```python
from build123d import *

# Parameters (mm, degrees)
FILLET1_R = 10


with BuildPart() as part:
    # Sketch1 → Revolve1 (revolve)
    with BuildSketch(Plane.XY, mode=Mode.PRIVATE) as revolve1_sk:
        Polygon((37.5, 42.257268448), (13.285767388, 0.316987298), (13.285767388, -0.683012702), (20.059447639, -25.962731552), (22.13, -25.962731552), (15.249019056, -0.282561065), (25.375644347, 17.257268448), (38.71, 17.257268448), (38.71, 42.257268448), align=None)
    revolve(revolve1_sk.sketch.rotate(Axis((0, 0, 0), (0, -1, 0)), 90), axis=Axis((0, 0, 0), (0, -1, 0)))

    # Fillet1
    fillet1_edges = [part.edges().sort_by_distance(p)[0] for p in [
        (0, 17.257268448, -25.375644347),
        (0, -0.282561065, -15.249019056),
    ]]
    fillet(fillet1_edges, radius=FILLET1_R)


solid = part.part
```
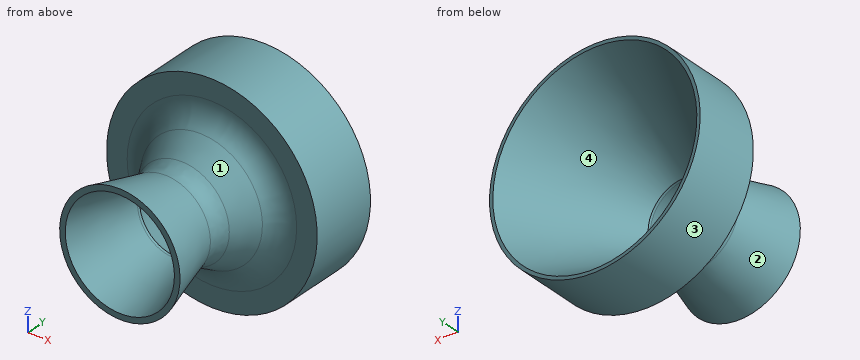
Input: part model. Units: mm. Frame: model coordinates. Face numbers are marked on the shaded views. Give positions to 0.01 mm unless a question says otherwise; leave off trailing zeros. Order: outer loops, then holes, each group sorted by start corner. A loop starts at its lowest first (then second) coordinate and runs counter-clockwise, first axis right, second up. Notation, with made-up numbers: (21.5, -29) - (61.5, -29) arc R8 cw to (61.5, -21) - close; hole circle Ø3 at (-11, 55.5). An arc over 180 degrees is marked (long way). One line per item, written item: value.
1. Pin query (flat end, axial travel): pin 1 Ø8 at (x, y) = (11.5, 16.5) entering from -Z; pin 2 Ø1 at (x, z) = (-8, 30.5) entering from -Y; pin 3 Ø2 at (x, z) = (-24, 2) entering from -Y. Return the tip coordinate at first contact, or that it passes through.
Determined:
pin 1: z = -37.96
pin 2: y = 17.26
pin 3: y = 13.17
2. Cut plane A-A, the plane y = 7.5. Output: boundary loops of the cut face in (x, z).
Determined:
outline: circle Ø39.48 at (0, 0); hole circle Ø34.87 at (0, 0)
3. Draft query along Y for the marked faces 1, 2, 3 and 4. Return one class per face: released by +Y, released by -Y, zero draft, split by the parting line, or undercut.
Determined:
face 1: undercut
face 2: undercut
face 3: zero draft
face 4: released by +Y
4. Cut plane B-B, the plane y = 22.5. Output: boundary loops of the cut face in (x, z).
Determined:
outline: circle Ø77.42 at (0, 0); hole circle Ø52.19 at (0, 0)
5. Line query: probe 1 along Z at (x, y) = (5.5, 11.5); probe 2 along Z at (x, y) = (2, -0.5); probe 3 along X at (y, z) = (-21, -4). Output: solid intervals per line, ascending.
Determined:
probe 1: -21.35 to -18.96, 18.96 to 21.35
probe 2: -15.93 to -13.13, 13.13 to 15.93
probe 3: -20.41 to -18.3, 18.3 to 20.41
